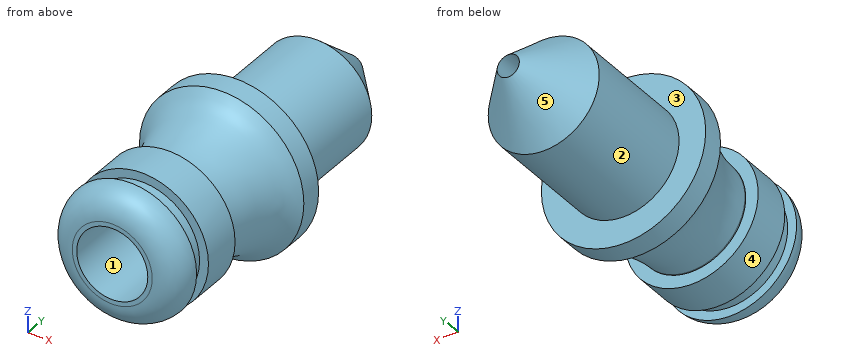
from build123d import *

# Parameters (mm, degrees)
F0_W = 2.25
F0_H = 10.4924628735
F2_R = 2.99999


# Not quite as in the source:
# - a fillet or chamfer is up to 0.001 mm smaller than in the source, because OpenCascade refuses the exact size


with BuildPart() as f1:
    # F0 (on Top) → F1 (revolve)
    with BuildSketch(Plane.XY):
        with BuildLine():
            Line((4, 10), (4, 0))
            Line((4, 0), (7.5, 0))
            Line((7.5, 0), (7.5, 3))
            Line((7.5, 3), (6.5, 3))
            Line((6.5, 3), (6.5, 5))
            Line((6.5, 5), (7.5, 5))
            Line((7.5, 5), (7.5, 9.5))
            Line((7.5, 9.5), (6.1, 9.5))
            add(Edge.make_bspline(
                [(6.1, 9.5), (6.0997806749, 9.542689319), (6.0997821122, 9.585377965), (6.1, 9.6280611679)],
                knots=[0, 0, 0, 0, 0.0093487262, 0.0093487262, 0.0093487262, 0.0093487262], degree=3))
            add(Edge.make_bspline(
                [(6.1, 9.6280611679), (6.1147869444, 12.5247545063), (7.6944598018, 17.0085980566), (8.4188714562, 17.7962221352), (9.25, 18.5)],
                knots=[0.0093487262, 0.0093487262, 0.0093487262, 0.0093487262, 0.6437995433, 1, 1, 1, 1], degree=3))
            Line((9.25, 18.5), (9.25, 21))
            Line((9.25, 21), (6.25, 21))
            Line((6.25, 21), (6.25, 24))
            Line((6.25, 24), (4, 24))
            Line((4, 24), (4, 10))
        make_face()
        with Locations((5.125, 29.2462314367)):
            Rectangle(F0_W, F0_H)
        Polygon((1.25, 37.7924628735), (4, 34.4924628735), (6.25, 34.4924628735), (1.25, 40.4924628735), align=None)
        with BuildLine():
            Line((6.1, 9.5), (6.1, 9.6280611679))
            add(Edge.make_bspline(
                [(6.1, 9.5), (6.0997806749, 9.542689319), (6.0997821122, 9.585377965), (6.1, 9.6280611679)],
                knots=[0, 0, 0, 0, 0.0093487262, 0.0093487262, 0.0093487262, 0.0093487262], degree=3))
        make_face()
    revolve(axis=Axis((0, 14.3348099664, 0), (0, 1, 0)))

    # F2 (radius 3 in the source; OpenCascade refuses exactly that, so slightly less here)
    f2_edges = [f1.edges().sort_by_distance(p)[0] for p in [
        (-7.5, 0, 0),
    ]]
    fillet(f2_edges, radius=F2_R)


solid = f1.part
Check sheet for the modelled part. Datum: model origin and axes. Units: mm. Face numbers are marked on the shaded views. A direction names the side the tool comes from. Give positions to 0.01 mm unless a question says otherwise; leave off trailing zeros. Order: outer loops, then holes, each group sorted by start corner. A loop starts at its lowest first (then second) coordinate and runs counter-clockwise, first axis right, second up. Notation, with made-up numbers: (49.5, -33) - (67.5, -33) arc R25 ccw to (67.5, -19) - close; hole circle Ø1 at (-38, 22). An arc over 180 degrees is marked (long way). Answer as CSV lines item,"result".
1. Mould release check, pull along X, two halves, no side actions. Record for the marked faces 1, 2 and 3: released by +X, released by -X, zero draft, split by the parting line, or undercut.
Result sheet:
face 1,"undercut"
face 2,"split by the parting line"
face 3,"zero draft"
2. Section check A-A (y = 21.5). Record the boundary of the cut face in (x, z).
Result sheet:
outline,"circle Ø12.5 at (0, 0); hole circle Ø8 at (0, 0)"
3. Go/stop test with flat-tipped pins: P1, Ø6, axis at x = 3, y = 35.5, coming from the +Z side; P2, Ø3, axis at x = -7, z = 2, coming from the +Y side; P3, Ø5, axis at y = 23, z = 3.5, coming from the -X side; P4, Ø1.5, axis at x = 0, z = 0, coming from the -Y side. Record where each tip stops, or that it passes through.
Result sheet:
P1,"z = 6.25"
P2,"y = 35.06"
P3,"x = -9.03"
P4,"through"
4. Section check B-B (y = 38.5). Record the boundary of the cut face in (x, z).
Result sheet:
outline,"circle Ø5.82 at (0, 0); hole circle Ø2.5 at (0, 0)"
5. Tool access check on the marked faces 4 and 5. Record the directions out of +Z, -Z, +X, -X, +Y, -Y that give a thin tool (end or side, any length) a straight path to the whole face; none if there is none.
Result sheet:
face 4,"-Y"
face 5,"+Y"
6. Scan lines: probe 1 along Z at (x, y) = (0, 20.5); probe 2 along Z at (x, y) = (0, 27.5); probe 3 along X at (y, z) = (31.5, -0.5). Record each from-to range of solid material in increasing order. Write a range as from..to.
Result sheet:
probe 1,"-9.25..-4, 4..9.25"
probe 2,"-6.25..-4, 4..6.25"
probe 3,"-6.23..-3.97, 3.97..6.23"
